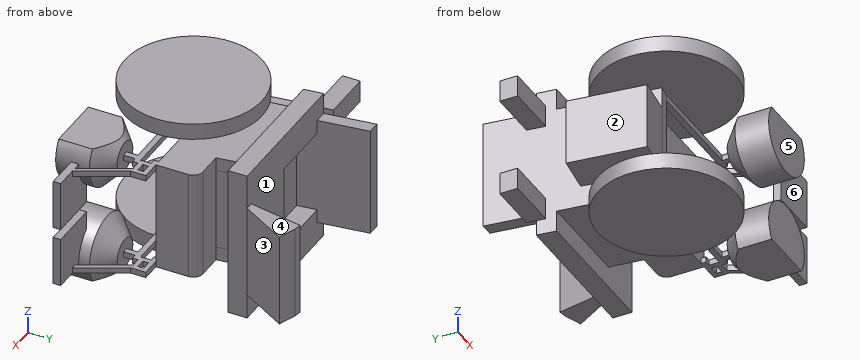
from build123d import *

# Parameters (mm, degrees)
BOSS_EXTRUDE1_DEPTH       = 30
BOSS_EXTRUDE1_DEPTH_BACK  = 55
SKETCH1_R                 = 360.2
BOSS_EXTRUDE2_DEPTH       = 55
BOSS_EXTRUDE2_DEPTH_BACK  = 30
SKETCH2_R                 = 360.2
BOSS_EXTRUDE3_DEPTH       = 10
BOSS_EXTRUDE6_DEPTH       = 575.8
BOSS_EXTRUDE33_DEPTH      = 400
BOSS_EXTRUDE33_DEPTH_BACK = 400
SKETCH25_W                = 366.7
SKETCH25_H                = 100
SKETCH5_W                 = 450
SKETCH5_H                 = 72
BOSS_EXTRUDE7_DEPTH       = 367.981167426
SKETCH8_W                 = 49.2
SKETCH8_H                 = 29.2
BOSS_EXTRUDE13_DEPTH      = 30
SKETCH19_R                = 177.8
BOSS_EXTRUDE22_DEPTH      = 270.2
CHAMFER1_SIZE             = 100
CHAMFER1_SIZE2            = 93.251508614
BOSS_EXTRUDE27_DEPTH      = 30
BOSS_EXTRUDE20_DEPTH      = 260
BOSS_EXTRUDE28_START      = 30
SKETCH23_W                = 30
SKETCH23_H                = 60
SKETCH23_W_2              = 49.2
SKETCH23_H_2              = 25.4
SKETCH23_W_3              = 25.4
BOSS_EXTRUDE28_DEPTH      = 30
SKETCH24_R                = 177.8
BOSS_EXTRUDE29_DEPTH      = 270.2
CHAMFER2_SIZE             = 100
CHAMFER2_SIZE2            = 93.251508614
BOSS_EXTRUDE30_DEPTH      = 30
BOSS_EXTRUDE31_DEPTH      = 260
BOSS_EXTRUDE18_START      = -83.975
BOSS_EXTRUDE18_DEPTH      = 113.975
BOSS_EXTRUDE19_START      = -30
BOSS_EXTRUDE19_DEPTH      = 113.975
BOSS_EXTRUDE32_START      = -575.8
BOSS_EXTRUDE32_DEPTH      = 575.8
BOSS_EXTRUDE34_REACH      = 1588.441
SKETCH26_W                = 184.1
SKETCH26_H                = 100
SKETCH27_W                = 350
SKETCH27_H                = 400
BOSS_EXTRUDE35_DEPTH      = 200
BOSS_EXTRUDE36_START      = -130
BOSS_EXTRUDE36_DEPTH      = 490
FILLET3_R                 = 50
SKETCH30_W                = 2623.123535912
SKETCH30_H                = 2420.43733062
CUT_EXTRUDE1_DEPTH        = 1934.451296391
SKETCH31_W                = 2584.765961417
SKETCH31_H                = 1858.147621016
CUT_EXTRUDE2_DEPTH        = 1913.404602985


# Read off the part's stored shape, not the designer's step: Boss-Extrude18, Boss-Extrude19, Boss-Extrude32
with BuildPart() as part:
    # Sketch1 → Boss-Extrude1 (new, two sides: drawn at the far end of the back side and taken through both)
    with BuildSketch(Plane.XY.offset(-BOSS_EXTRUDE1_DEPTH_BACK)):
        with Locations((330.2, 330.2)):
            Circle(SKETCH1_R)
    extrude(amount=BOSS_EXTRUDE1_DEPTH + BOSS_EXTRUDE1_DEPTH_BACK)



with BuildPart() as body_2:
    # Sketch2 → Boss-Extrude2 (new, two sides: drawn at the far end of the back side and taken through both)
    with BuildSketch(Plane.XY.offset(-685.8).offset(-BOSS_EXTRUDE2_DEPTH_BACK)):
        with Locations((330.2, 330.2)):
            Circle(SKETCH2_R)
    extrude(amount=BOSS_EXTRUDE2_DEPTH + BOSS_EXTRUDE2_DEPTH_BACK)


with BuildPart() as part_1:
    add(part.part)

    add(body_2.part)  # Boss-Extrude3 merges body 2
    # 3DSketch2 → Boss-Extrude3 (add)
    with BuildSketch(Plane(origin=(330.2, 460, -630.8), x_dir=(0.5893057409504111, 0, 0.807910108664873), z_dir=(0, -1, 0))):
        Polygon((465.194640569, 339.322245639), (0, 0), (247.508411199, -339.322245639), (712.703051768, 0), align=None)
        Polygon((-38.304873162, 52.514157063), (0, 0), (465.194640569, 339.322245639), (426.889767407, 391.836402702), align=None)
    extrude(amount=-BOSS_EXTRUDE3_DEPTH)

    # Sketch4 → Boss-Extrude6 (add)
    with BuildSketch(Plane(origin=(0, -170.8, -630.8), x_dir=(1, 0, 0), z_dir=(0, 0, 1))):
        Polygon((208.828935151, 1364.6), (330.2, 501), (265.832575532, 491.953748438), (143.190142937, 1364.6), align=None)
    extrude(amount=BOSS_EXTRUDE6_DEPTH)

    # Sketch5 → Boss-Extrude7 (add, along a direction that is not the sketch's normal)
    with BuildSketch(Plane(origin=(0, 470, 0), x_dir=(1, 0, 0), z_dir=(0, 1, 0))):
        with Locations((535.552391309, 91)):
            Rectangle(SKETCH5_W, SKETCH5_H)
        with Locations((535.552391309, 594.8)):
            Rectangle(SKETCH5_W, SKETCH5_H)
    extrude(amount=BOSS_EXTRUDE7_DEPTH, dir=(-0.13917310096006222, 0.9902680687415708, 0))

    # Sketch8 → Boss-Extrude13 (add)
    with BuildSketch(Plane(origin=(0, 0, -630.8), x_dir=(-1, 0, 0), z_dir=(0, 0, -1))):
        Polygon((-1014.4, 360.2), (-939.8, 360.2), (-939.8, 330.2), (-914.4, 330.2), (-914.4, 270.2), (-884.4, 270.2), (-884.4, 330.2), (-330.2, 330.2), (-325.983774959, 360.2), (-914.4, 360.2), (-914.4, 414.8), (-884.4, 414.8), (-884.4, 440.2), (-1014.4, 440.2), align=None)
        with Locations((-964.4, 400.2)):
            Rectangle(SKETCH8_W, SKETCH8_H, mode=Mode.SUBTRACT)
    extrude(amount=-BOSS_EXTRUDE13_DEPTH)

    # Sketch19 → Boss-Extrude22 (add)
    with BuildSketch(Plane.XZ.offset(-270.2)):
        with Locations(Location((899.4, -615.8, 0), (0, 0, 90))):
            Circle(SKETCH19_R)
    extrude(amount=BOSS_EXTRUDE22_DEPTH)

    # Chamfer1
    chamfer1_edges = [part_1.edges().sort_by_distance(p)[0] for p in [
        (899.4, 270.2, -793.6),
    ]]
    chamfer1_side = [part_1.faces().sort_by_distance(p)[0] for p in [
        (899.4, 270.2, -788.571056572),
    ]]
    chamfer(chamfer1_edges, length=CHAMFER1_SIZE, length2=CHAMFER1_SIZE2, reference=chamfer1_side[0])

    # Sketch8<7> → Boss-Extrude27 (add)
    with BuildSketch(Plane(origin=(0, 0, -630.8), x_dir=(-1, 0, 0), z_dir=(0, 0, -1))):
        Polygon((-1014.4, 360.2), (-1140.7, 120.65), (-1115.3, 120.65), (-989, 360.2), align=None)
    extrude(amount=-BOSS_EXTRUDE27_DEPTH)

    # Sketch8<4> → Boss-Extrude20 (add)
    with BuildSketch(Plane(origin=(0, 0, -630.8), x_dir=(-1, 0, 0), z_dir=(0, 0, -1))):
        Polygon((-1256.425, 81.125), (-1256.425, 120.65), (-1140.7, 120.65), (-1115.3, 120.65), (-999.575, 120.65), (-999.575, 81.125), align=None)
    extrude(amount=-BOSS_EXTRUDE20_DEPTH)

    # Sketch23 → Boss-Extrude28 (add)
    with BuildSketch(Plane(origin=(0, 0, -55), x_dir=(-1, 0, 0), z_dir=(0, 0, -1)).offset(BOSS_EXTRUDE28_START)):
        with BuildLine():
            Line((-330.2, 360.2), (-689.148519986, 360.2))
            ThreePointArc((-689.148519986, 360.2), (-690.086993999, 345.213046012), (-690.4, 330.2))
            Line((-690.4, 330.2), (-330.2, 330.2))
            Line((-330.2, 330.2), (-330.2, 360.2))
        make_face()
        with BuildLine():
            Line((-914.4, 360.2), (-939.8, 360.2))
            Line((-939.8, 360.2), (-939.8, 330.2))
            Line((-939.8, 330.2), (-914.4, 330.2))
            Line((-914.4, 330.2), (-884.4, 330.2))
            Line((-884.4, 330.2), (-690.4, 330.2))
            ThreePointArc((-690.4, 330.2), (-690.086993999, 345.213046012), (-689.148519986, 360.2))
            Line((-689.148519986, 360.2), (-914.4, 360.2))
        make_face()
        with Locations((-899.4, 300.2)):
            Rectangle(SKETCH23_W, SKETCH23_H)
        Polygon((-939.8, 385.6), (-939.8, 360.2), (-914.4, 360.2), (-914.4, 414.8), (-914.4, 440.2), (-939.8, 440.2), (-939.8, 414.8), align=None)
        with Locations((-964.4, 372.9)):
            Rectangle(SKETCH23_W_2, SKETCH23_H_2)
        with Locations((-964.4, 427.5)):
            Rectangle(SKETCH23_W_2, SKETCH23_H_2)
        Polygon((-1014.4, 440.2), (-1014.4, 385.6), (-989, 385.6), (-989, 414.8), (-989, 440.2), align=None)
        with Locations((-1001.7, 372.9)):
            Rectangle(SKETCH23_W_3, SKETCH23_H_2)
        Polygon((-325.983774959, 360.2), (-330.2, 360.2), (-330.2, 330.2), align=None)
        with Locations((-899.4, 427.5)):
            Rectangle(SKETCH23_W, SKETCH23_H_2)
    extrude(amount=-BOSS_EXTRUDE28_DEPTH)

    # Sketch24 → Boss-Extrude29 (add)
    with BuildSketch(Plane(origin=(0, 270.2, 0), x_dir=(-1, 0, 0), z_dir=(0, -1, 0))):
        with Locations(Location((-899.4, 70, 0), (0, 0, 270))):
            Circle(SKETCH24_R)
    extrude(amount=BOSS_EXTRUDE29_DEPTH)

    # Chamfer2
    chamfer2_edges = [part_1.edges().sort_by_distance(p)[0] for p in [
        (899.4, 270.2, -247.8),
    ]]
    chamfer2_side = [part_1.faces().sort_by_distance(p)[0] for p in [
        (899.4, 270.2, -242.771056572),
    ]]
    chamfer(chamfer2_edges, length=CHAMFER2_SIZE, length2=CHAMFER2_SIZE2, reference=chamfer2_side[0])

    # Sketch23<10> → Boss-Extrude30 (add)
    with BuildSketch(Plane(origin=(0, 0, -55), x_dir=(-1, 0, 0), z_dir=(0, 0, -1))):
        Polygon((-1014.4, 360.2), (-1140.7, 120.65), (-1115.3, 120.65), (-989, 360.2), align=None)
    extrude(amount=BOSS_EXTRUDE30_DEPTH)

    # Sketch23<12> → Boss-Extrude31 (add)
    with BuildSketch(Plane(origin=(0, 0, -55), x_dir=(-1, 0, 0), z_dir=(0, 0, -1))):
        Polygon((-1256.425, 81.125), (-1256.425, 120.65), (-1140.7, 120.65), (-1115.3, 120.65), (-999.575, 120.65), (-999.575, 81.125), align=None)
    extrude(amount=BOSS_EXTRUDE31_DEPTH)

    # Boss-Extrude18 outline → Boss-Extrude18 (add)
    with BuildSketch(Plane(origin=(0, 0, -630.8), x_dir=(-1, 0, 0), z_dir=(0, 0, -1)).offset(BOSS_EXTRUDE18_START)):
        Polygon((93.839496852, 982.025), (-172.953178206, 982.025), (-186.160503148, 888.05), (93.839496852, 888.05), align=None)
    extrude(amount=BOSS_EXTRUDE18_DEPTH)

    # Boss-Extrude19 outline → Boss-Extrude19 (add)
    with BuildSketch(Plane(origin=(0, 0, -55), x_dir=(-1, 0, 0), z_dir=(0, 0, -1)).offset(BOSS_EXTRUDE19_START)):
        Polygon((93.839496852, 982.025), (-172.953178206, 982.025), (-186.160503148, 888.05), (93.839496852, 888.05), align=None)
    extrude(amount=BOSS_EXTRUDE19_DEPTH)

    # Boss-Extrude32 outline → Boss-Extrude32 (add)
    with BuildSketch(Plane(origin=(0, 0, -630.8), x_dir=(-1, 0, 0), z_dir=(0, 0, -1)).offset(BOSS_EXTRUDE32_START)):
        with BuildLine():
            Line((-750.2, 460), (-750.2, 470))
            Line((-750.2, 470), (-310.552391309, 470))
            Line((-310.552391309, 470), (-283.793416382, 660.4))
            Line((-283.793416382, 660.4), (-474.11664254, 660.4))
            ThreePointArc((-474.11664254, 660.4), (-378.928501989, 687.088740497), (-280.069849034, 686.894558361))
            Line((-280.069849034, 686.894558361), (-259.339311143, 834.4))
            Line((-259.339311143, 834.4), (-709.339311143, 834.4))
            Line((-709.339311143, 834.4), (-733.793416381, 660.4))
            Line((-733.793416381, 660.4), (-914.4, 660.4))
            Line((-914.4, 660.4), (-914.4, 440.2))
            Line((-914.4, 440.2), (-314.740508183, 440.2))
            Line((-314.740508183, 440.2), (-311.957799656, 460))
            Line((-311.957799656, 460), (-750.2, 460))
        make_face()
    extrude(amount=BOSS_EXTRUDE32_DEPTH)



with BuildPart() as body_2_2:
    # Sketch25 → Boss-Extrude33 (new, two sides: drawn at the far end of the back side and taken through both)
    with BuildSketch(Plane.XY.offset(-342.9).offset(-BOSS_EXTRUDE33_DEPTH_BACK)):
        with Locations((760.189311143, 884.4)):
            Rectangle(SKETCH25_W, SKETCH25_H)
    extrude(amount=BOSS_EXTRUDE33_DEPTH + BOSS_EXTRUDE33_DEPTH_BACK)


with BuildPart() as part_2:
    add(part_1.part)

    add(body_2_2.part)  # Boss-Extrude34 merges body 2 2
    # Boss-Extrude34: up to this plane
    boss_extrude34_end = Plane(origin=(143.190142937, 1193.8, 837.459616456), z_dir=(0.9902680687415708, 0.1391731009600622, 0))
    # Sketch26 → Boss-Extrude34 (add, up to the surface)
    with BuildSketch(Plane.ZY.offset(-576.839311143), mode=Mode.PRIVATE) as boss_extrude34_sk1:
        with Locations((-34.95, 884.4)):
            Rectangle(SKETCH26_W, SKETCH26_H)
    boss_extrude34_tool1 = split(extrude(boss_extrude34_sk1.sketch, amount=BOSS_EXTRUDE34_REACH, mode=Mode.PRIVATE), bisect_by=boss_extrude34_end, keep=Keep.BOTH, mode=Mode.PRIVATE)
    add(boss_extrude34_tool1.solids().sort_by_distance((576.839311, 884.4, -34.95))[0])
    # Sketch26 → Boss-Extrude34 (add, up to the surface)
    with BuildSketch(Plane.ZY.offset(-576.839311143), mode=Mode.PRIVATE) as boss_extrude34_sk2:
        with Locations((-650.85, 884.4)):
            Rectangle(SKETCH26_W, SKETCH26_H)
    boss_extrude34_tool2 = split(extrude(boss_extrude34_sk2.sketch, amount=BOSS_EXTRUDE34_REACH, mode=Mode.PRIVATE), bisect_by=boss_extrude34_end, keep=Keep.BOTH, mode=Mode.PRIVATE)
    add(boss_extrude34_tool2.solids().sort_by_distance((576.839311, 884.4, -650.85))[0])

    # Sketch27 → Boss-Extrude35 (add)
    with BuildSketch(Plane(origin=(304.944608977, 42.857169884, 0), x_dir=(0, 0, 1), z_dir=(-0.9902680687415708, -0.13917310096006216, 0))):
        with Locations((-342.9, 481.031558361)):
            Rectangle(SKETCH27_W, SKETCH27_H)
    extrude(amount=BOSS_EXTRUDE35_DEPTH)

    # Sketch29 → Boss-Extrude36 (add)
    with BuildSketch(Plane(origin=(0, 0, -742.9), x_dir=(-1, 0, 0), z_dir=(0, 0, -1)).offset(BOSS_EXTRUDE36_START)):
        Polygon((-1083.539311143, 1176.88711306), (-992.16080089, 1210.146170843), (-943.539311143, 934.4), align=None)
        Polygon((-992.16080089, 1210.146170843), (-943.539311143, 934.4), (-902.922246668, 934.4), (-952.768490769, 1217.09209795), align=None)
    extrude(amount=-BOSS_EXTRUDE36_DEPTH)

    # Fillet3
    fillet3_edges = [part_2.edges().sort_by_distance(p)[0] for p in [
        (914.4, 660.4, -342.9),
    ]]
    fillet(fillet3_edges, radius=FILLET3_R)

    # Sketch30 → Cut-Extrude1 (cut, through all)
    with BuildSketch(Plane.XY.offset(30)):
        with Locations((451.826678709, -519.81866531)):
            Rectangle(SKETCH30_W, SKETCH30_H)
    extrude(amount=CUT_EXTRUDE1_DEPTH, mode=Mode.SUBTRACT)

    # Sketch31 → Cut-Extrude2 (cut, through all)
    with BuildSketch(Plane(origin=(0, 0, -715.8), x_dir=(-1, 0, 0), z_dir=(0, 0, -1))):
        with Locations((-741.050727566, -238.673810508)):
            Rectangle(SKETCH31_W, SKETCH31_H)
    extrude(amount=CUT_EXTRUDE2_DEPTH, mode=Mode.SUBTRACT)


solid = part_2.part
Verification items for the finished model (mm, model axes). Face numbers are marked on the shaded views. A direction names the side the tool comes from. Give positions to 0.01 mm unless a question says otherwise; leave off trailing zeros. Write each loop counter-clockwise with the first axis right and the second up, starting at its lowest first coordinate (ties: lowest second). Pieces come first, ordered by that corner, then holes. Notation, with made-up numbers: (63, 11.5) - (89, 11.5) arc R23 cw to (89, 27.5) - close; hole circle Ø9 at (3.25, 38). An arc over 180 degrees is marked (long way). Answer as CSV lines item,"result". Start each with the question number.
1. Draft check along Y on the marked faces 1, 2 and 3. Enter one of: pulls with the +Y half, pulls with the -Y half, needs draft (parallel to the pull), parting line crosses it, or undercut.
2. Sectioned sample at A-A (y = 1029). Record the boundary of the cut face in (x, z).
3. Set-up check for the marked faces 4, 5 and 6: record each of +Z, -Z, +X, -X, +Y, -Y from which the full face is reachable in a straight line by a thin tool's end or side.
4. Thickness scan on line 1 (Z direction, x = 660, y = 389); line 2 (Y direction, x = 793.5, z = -499.5); line 3 (Y direction, x = 763, z = -384.5). Record the ranges inside material, lowest first.
5. Depth check by flat-ended pin: pin 1 (12 mm diameter, centred on x = 761.5, z = -41, fed in from +Y); pin 2 (1.5 mm diameter, centred on y = 894, z = -373.5, fed in from +X); pin 3 (24 mm diameter, centred on x = 968.5, z = -64, fed in from -Y). Enter the tip coordinate at first touch or a pass-through.
6. Sectioned sample at C-C (y = 780). Record the boundary of the cut face in (x, z).
Derived:
1,face 1,"pulls with the +Y half"
1,face 2,"pulls with the -Y half"
1,face 3,"undercut"
2,outline,"(166.35, -630.8) - (231.99, -630.8) - (231.99, -55) - (166.35, -55) - close; (919.6, -612.9) - (998.16, -612.9) - (998.16, -122.9) - (919.6, -122.9) - close"
3,face 4,"+Z, +X, +Y"
3,face 5,"+Z, -Z, +X, -Y"
3,face 6,"+X, -Y"
4,line 1,"-715.8 to -630.8, -55 to 30"
4,line 2,"0 to 196.07, 440.2 to 660.4, 834.4 to 934.4"
4,line 3,"440.2 to 660.4, 834.4 to 934.4"
5,pin 1,"y = 934.4"
5,pin 2,"x = 943.54"
5,pin 3,"y = 0"
6,outline,"(201.35, -630.8) - (716.98, -630.8) - (716.98, -55) - (201.35, -55) - close"
